Build history of the part. All positions in model axes, mm. A direction names the side the tool comes from. Give positions to 0.01 mm unless a question says otherwise; leave off trailing zeros. Loops run counter-clockwise (first coordinate to the right, second up) from the corner with the lowest first, then second, coordinate; pieces in that order, holes last. Notation, with made-up numbers: (-0.75, 69.5) -> (4.25, 69.5) arc R14 ccw to (4.25, 73.5) -> close; hole circle Ø1 at (44.25, -16). An arc over 180 degrees is marked (long way). Answer in a Markdown table with one row per item. Add a question column.
from build123d import *

# Parameters (mm, degrees)
SKETCH2_W          = 0.5
SKETCH2_H          = 5.643439565
CUT_EXTRUDE1_DEPTH = 10
CIRPATTERN1_COUNT  = 4


with BuildPart() as part:
    # Sketch1 → Revolve1 (revolve)
    with BuildSketch(Plane.XY):
        with BuildLine():
            Line((0, 5.741657387), (0, 4))
            ThreePointArc((0, 4), (3.373565783, 2.149198433), (3.625231148, -1.690473047))
            Line((3.625231148, -1.690473047), (4.078385042, -1.901782178))
            ThreePointArc((4.078385042, -1.901782178), (4.333692417, 1.212068493), (2.5, 3.741657387))
            Line((2.5, 3.741657387), (2.5, 5.741657387))
            Line((2.5, 5.741657387), (0, 5.741657387))
        make_face()
    revolve(axis=Axis((0, 5.741657387, 0), (0, -1, 0)))

    # Sketch2 → Cut-Extrude1 (cut)
    with BuildSketch(Plane.XY):
        with Locations((0, 0.919937604)):
            Rectangle(SKETCH2_W, SKETCH2_H)
    cut_extrude1 = extrude(amount=-CUT_EXTRUDE1_DEPTH, mode=Mode.SUBTRACT)

    # CirPattern1: Cut-Extrude1 ×4 about axis
    cirpattern1_axis = Axis((0, 0, 0), (0, 1, 0))
    for i in range(1, CIRPATTERN1_COUNT):
        add(cut_extrude1.rotate(cirpattern1_axis, i * 360 / CIRPATTERN1_COUNT), mode=Mode.SUBTRACT)


solid = part.part
(1) Two-plate mould, pull along X, no slides. Class faces 3 (the flat face through (-4, 1.1, 0.25)), 4 (the flat face through (0.25, 1.1, -4)), 5 (the cylindrical face through (-0.54, 4.76, -2.44)): released by +X, released by -X, zero draft, split by the parting line, or undercut.
(2) Wall check: line 1 along Z through (x, y) = (3, 0.5); line 2 along X through (y, z) = (1.75, -1); line 3 along Z through (x, y) = (3.5, 0.5). Give the ranges that are in metal, low to high. Write a range as from..to.
(3) Saw through at C-C, the plane z = 0. List the corners of the cut face in (x, y), then the cut area to 3 significant figures.
(4) Saw through at D-D, the plane y = 0.25. List the corners of the cut face in (x, z), then the cut area to 3 significant figures.
(5) 3-axis set-ups, long thin cutter, end or side, ignore diameter. For faces 1 (the flat face through (0, 5.742, 0)), 2 (the conical face through (2.717, -1.774, 2.663)): which of +Z, -Z, +X, -X, +Y, -Y reach the whole face in a straight line?
(6) Saw through at B-B, the plane y = 4.25. List the corners of the cut face in (x, z).
(7) Flat gauge pins, fed straight in: pin 1 Ø4 at (x, y) = (2, 1) entering from +Z; pin 2 Ø2.5 at (y, z) = (0, 2) entering from -X; pin 3 Ø4 at (x, y) = (2.5, 1.5) entering from -Z. Where does each tip first touch, or does it go through?
(8) Saw through at A-A, the plane y = 2.25. List the corners of the cut face in (x, z), then the cut area to 3 significant figures.
Worked answers:
| question | item | result |
|---|---|---|
| 1 | face 3 | zero draft |
| 1 | face 4 | undercut |
| 1 | face 5 | split by the parting line |
| 2 | line 1 | -3.32..-2.6, 2.6..3.32 |
| 2 | line 2 | -4.02..-3.46, 3.46..4.02 |
| 2 | line 3 | -2.78..-1.87, 1.87..2.78 |
| 3 | outline | (-2.5, 3.74) -> (-1.41, 3.74) arc R4 cw to (1.41, 3.74) -> (2.5, 3.74) -> (2.5, 5.74) -> (-2.5, 5.74) -> close |
| 3 | area | 9.51 mm^2 |
| 4 | outline | (-4.49, -0.25) arc R4.49 ccw to (-0.25, -4.49) -> (-0.25, -3.98) arc R3.99 cw to (-3.98, -0.25) -> close; (-4.49, 0.25) -> (-3.98, 0.25) arc R3.99 cw to (-0.25, 3.98) -> (-0.25, 4.49) arc R4.49 ccw to start; (0.25, -4.49) arc R4.49 ccw to (4.49, -0.25) -> (3.98, -0.25) arc R3.99 cw to (0.25, -3.98) -> close; (0.25, 3.98) arc R3.99 cw to (3.98, 0.25) -> (4.49, 0.25) arc R4.49 ccw to (0.25, 4.49) -> close |
| 4 | area | 12.3 mm^2 |
| 5 | face 1 | +Z, -Z, +X, -X, +Y |
| 5 | face 2 | -Y |
| 6 | outline | circle Ø5 at (0, 0) |
| 7 | pin 1 | z = 4.49 |
| 7 | pin 2 | x = -4.44 |
| 7 | pin 3 | z = -4.41 |
| 8 | outline | (-3.89, -0.25) arc R3.9 ccw to (-0.25, -3.89) -> (-0.25, -3.3) arc R3.31 cw to (-3.3, -0.25) -> close; (-3.89, 0.25) -> (-3.3, 0.25) arc R3.31 cw to (-0.25, 3.3) -> (-0.25, 3.89) arc R3.9 ccw to start; (0.25, -3.89) arc R3.9 ccw to (3.89, -0.25) -> (3.3, -0.25) arc R3.31 cw to (0.25, -3.3) -> close; (0.25, 3.3) arc R3.31 cw to (3.3, 0.25) -> (3.89, 0.25) arc R3.9 ccw to (0.25, 3.89) -> close |
| 8 | area | 12.2 mm^2 |
